Can you work these out from the drawing? Everything is in mm from the part's minimum corner. Coordinates: 2 decimals unless noted, no trailing zeros. Order: outer loops, then holes, each group sorted by start corner. A loop starts at its lowest first (then second) coordinate and runs counter-clockwise, first axis right, second up. Notation, with made-up numbers: (-12, 53.5) -> (46, 53.5) arc R17 cw to (46, 82.5) -> close; hole circle Ø5 at (65, 76.25). An arc over 180 degrees is marked (long way). Put each result on its own line as item: value. Start each with the question number.
Q1. Please list where these lines run through material, in increasing order: line 1 along X through (y, z) = (2.2, 60); line 2 along Z through (x, y) = (46.5, 2.15) (1 decimal); line 3 along Z through (x, y) = (49, 0.8).
Q2. If we section it at D-D (y = 1.7): Count the separate pieces of the cut face and the enclosed holes in it, and give its area (3 significant figures).
Q3. If we section it at A-A (z = 60): Please give me the cut outline in (x, y).
Q4. If we section it at B-B (x = 48): Please give me the cut outline in (y, z).
Q5. Will these pins go through, and if not, where does the flat tip stop? pin 1 (1.5 mm diameter, centred on y = 1.5, z = 89.5, fed in from -X); pin 2 (0.9 mm diameter, centred on x = 86.5, y = 1, fed in from +Z); pin 3 (0.9 mm diameter, centred on x = 4.5, y = 2, fed in from +Z).
Q6. If we section it at C-C (z = 30): Please give me the cut outline in (x, y).
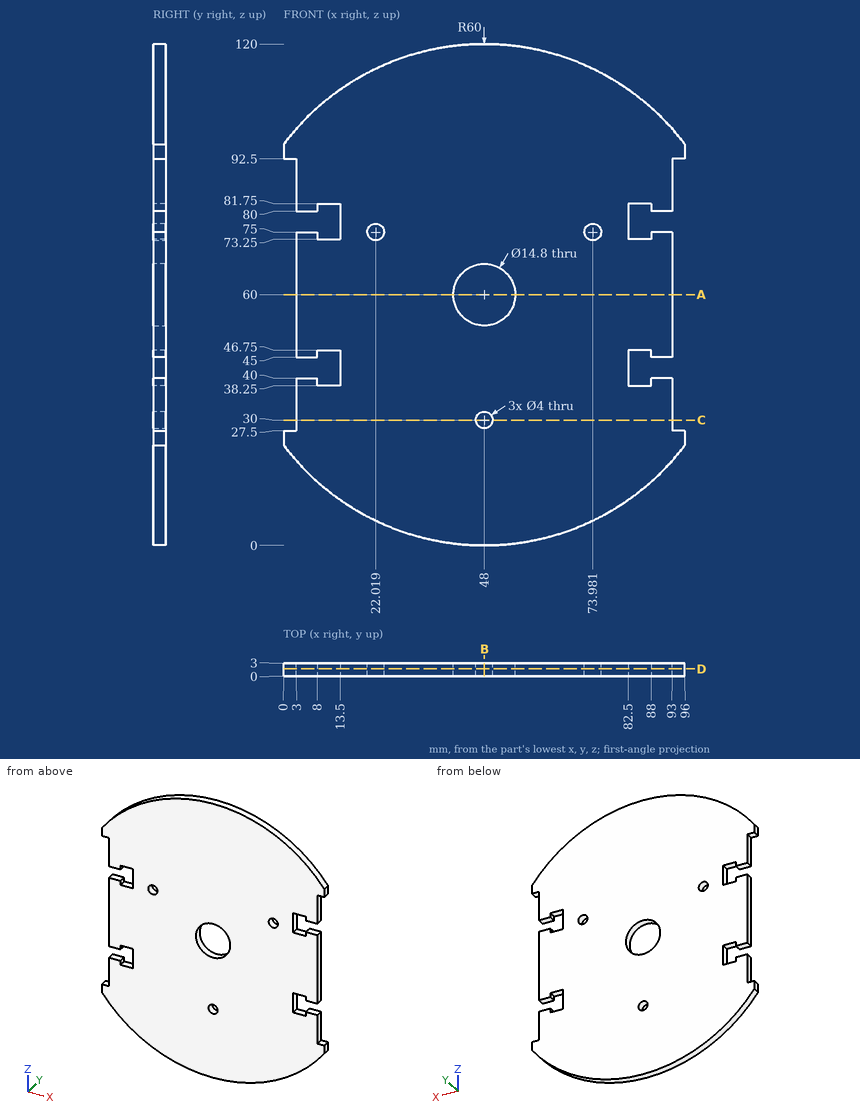
The answers:
1. line 1: 3 to 40.6, 55.4 to 93
1. line 2: 0 to 28.7, 31.3 to 52.8, 67.2 to 120
1. line 3: 0.01 to 28.27, 31.73 to 52.67, 67.33 to 119.99
2. separate pieces: 1
2. enclosed holes: 4
2. area: 9,250 mm^2
3. outline: (3, 0) -> (40.6, 0) -> (40.6, 3) -> (3, 3) -> close; (55.4, 0) -> (93, 0) -> (93, 3) -> (55.4, 3) -> close
4. outline: (0, 0) -> (3, 0) -> (3, 28) -> (0, 28) -> close; (0, 32) -> (3, 32) -> (3, 52.6) -> (0, 52.6) -> close; (0, 67.4) -> (3, 67.4) -> (3, 120) -> (0, 120) -> close
5. pin 1: x = 3
5. pin 2: z = 106.39
5. pin 3: z = 101.79
6. outline: (3, 0) -> (46, 0) -> (46, 3) -> (3, 3) -> close; (50, 0) -> (93, 0) -> (93, 3) -> (50, 3) -> close
